Build history of the part. All positions in model axes, mm. Give positions to 0.01 mm unless a question says otherwise; leave off trailing zeros. Order: outer loops, then holes, each group sorted by start corner. A loop starts at its lowest first (then second) coordinate and runs counter-clockwise, first axis right, second up. Notation, with made-up numbers: (87, 33) - (113, 33) arc R20 cw to (113, 72) - close; hole circle Ø8 at (-31.75, 38). An arc over 180 degrees is marked (long way). One line per item, written item: value.
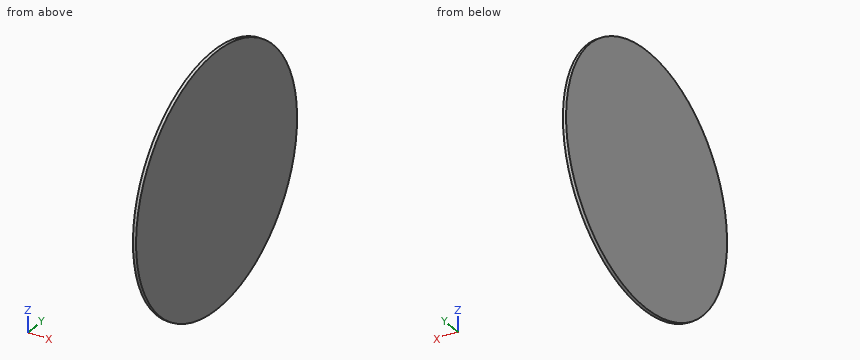
```python
from build123d import *

# Parameters (mm, degrees)
SKETCH1_R             = 40
BOSS_EXTRUDE1_DEPTH   = 1
SCALE1_SCALE          = 0.5
SCALE3_SCALE          = 0.625
BODY_MOVE_COPY4_ANGLE = 30
BODY_MOVE_COPY5_ANGLE = 30


with BuildPart() as part:
    # Sketch1 → Boss-Extrude1 (new body)
    with BuildSketch(Plane(origin=(0, 0, 0), x_dir=(0, 0, -1), z_dir=(1, 0, 0))):
        Circle(SKETCH1_R)
    extrude(amount=BOSS_EXTRUDE1_DEPTH)


with BuildPart() as part_1:
    # Scale1: scaled about (0.5, 0, 0)
    add(part.part.scale(SCALE1_SCALE).moved(Location((0.25, 0, 0))))


with BuildPart() as part_2:
    # Body-Move/Copy2: moved
    add(part_1.part.moved(Location((4.171055646, 0, 0))))


with BuildPart() as part_3:
    # Scale3: scaled about (4.671055646, 0, 0)
    add(part_2.part.scale(SCALE3_SCALE).moved(Location((1.751645867, 0, 0))))


with BuildPart() as part_4:
    # Body-Move/Copy4: read off the stored shape, not the designer's step
    # Body-Move/Copy4: moved
    add(part_3.part.moved(Location((-0.8605566, 0, -3.1693539))).rotate(Axis((0, 0, 0), (0, -1, 0)), BODY_MOVE_COPY4_ANGLE))


with BuildPart() as part_5:
    # Body-Move/Copy5: read off the stored shape, not the designer's step
    # Body-Move/Copy5: moved
    add(part_4.part.moved(Location((-0.3011634, 0, 2.7353489))).rotate(Axis((0, 0, 0), (0, 1, 0)), BODY_MOVE_COPY5_ANGLE))


solid = part_5.part
```
(1) Drill centre lines: line 1 (Z direction, x = 4.8, y = 3.75); line 2 (Y direction, x = 4.85, z = -10.25); line 3 (Z direction, x = 5, y = -9.5). Where is each one in solid material? Low to high.
Completed:
line 1: -12.57 to 11.27
line 2: -8.01 to 8.01
line 3: -8.77 to 7.47
(2) Slice it at B-B, the plane y = 2.25. Give the cut face in (x, z), and give its area (3 significant figures).
Completed:
outline: (4.76, -12.95) - (5.07, -12.95) - (5.07, 11.65) - (4.76, 11.65) - close
area: 7.68 mm²
(3) Slice it at A-A, the plane x = 5. Give the cut face in (y, z), and give its area (3 significant figures).
Completed:
outline: circle Ø25 at (0, -0.65)
area: 491 mm²
(4) Slice it at C-C, the plane z = 7.5. Give the cut face in (x, y).
Completed:
outline: (4.76, -9.48) - (5.07, -9.48) - (5.07, 9.48) - (4.76, 9.48) - close
